Autodesk Inventor part; units mm, degrees
ref_plane "YZ Plane" through (0, 0, 0) normal (1, 0, 0) x (0, 1, 0)
ref_plane "XZ Plane" through (0, 0, 0) normal (0, 1, 0) x (-1, 0, 0)
ref_plane "XY Plane" through (0, 0, 0) normal (0, 0, 1) x (1, 0, 0)
ref_plane "Work Plane1" through (0, 0, 0) normal (0, 0, 1) x (1, 0, 0)
sketch "Sketch1" plane through (0, 0, 0) normal (0, 0, 1) x (1, 0, 0)
  line L0 (10.1591, -5.9453) -> (35.8591, -5.9453)
  line L1 (35.8591, -5.9453) -> (35.8591, -11.7453)
  line L2 (35.8591, -11.7453) -> (10.1591, -11.7453)
  line L3 (10.1591, -11.7453) -> (10.1591, -5.9453)
  point P0 (0, 0)
  dimension "d0" = 25.7
  dimension "d2" = 5.8
extrude "Extrusion1" add sketch "Sketch1" along normal blind 13.2
chamfer "Chamfer1" distance 9.2 angle 45 1 edges at (10.1591, -8.8453, 13.2)
sketch "Sketch2" plane through (35.8591, -11.7453, 0) normal (1, 0, 0) x (0, 0, -1)
  line L0 (0, 5.8) -> (0, 0)
  line L1 (0, 5.8) -> (-13.2, 5.8)
  line L2 (-13.2, 0) -> (-13.2, 5.8)
  line L3 (0, 0) -> (-13.2, 0)
  line L4 (-12.8, 5.4) -> (-0.4, 5.4)
  line L5 (-0.4, 5.4) -> (-0.4, 0.4)
  line L6 (-0.4, 0.4) -> (-12.8, 0.4)
  line L7 (-12.8, 0.4) -> (-12.8, 5.4)
  point P0 (0, 11.7453)
  dimension "d8" = 0.4
extrude "Extrusion2" cut sketch "Sketch2" against normal blind 16 contours L4 L5 L6 L7
sketch "Sketch3" plane through (19.8591, -11.7453, 0) normal (1, 0, 0) x (0, 0, -1)
  line L0 (-12.8, 5.4) -> (-0.4, 5.4)
  line L1 (-12.8, 0.4) -> (-12.8, 5.4)
  line L2 (-0.4, 5.4) -> (-0.4, 0.4)
  line L3 (-12.4, 5) -> (-0.8, 5)
  line L4 (-0.8, 5) -> (-0.8, 3.6)
  line L5 (-0.8, 3.6) -> (-12.4, 3.6)
  line L6 (-12.4, 3.6) -> (-12.4, 5)
  point P0 (0, 11.7453)
  dimension "d11" = 0.4
  dimension "d12" = 0.4
  dimension "d13" = 0.4
  dimension "d14" = 1.4
extrude "Extrusion3" add sketch "Sketch3" along normal blind 16
properties part number "nanopc_t4_usb3"
The model under review builds one solid part; all positions refer to its coordinate system, in mm. A direction names the side the tool comes from. Round coordinates to 2 decimals unless told otherwise and drop trailing zeros. Order: outer loops, then holes, each group sorted by start corner. A loop starts at its lowest first (then second) coordinate and runs counter-clockwise, first axis right, second up. Notation, with made-up numbers: (-36.75, 72.5) -> (13.25, 72.5) arc R30 cw to (13.25, 95.5) -> close; hole circle Ø10 at (6, -25.5). An arc over 180 degrees is marked (long way). Use CSV: the item, a comma, the result in double quotes. Start each with the question number.
(1) Consider section A-A on x = 34.25. Write out the cut boundary in (y, z), and give its area (3 significant figures).
(2) Mouldability with a two-part tool opening along Z and no side actions: class faces 1 (the face through (23, -5.945, 7)), 2 (the face through (19.859, -9, 7)), 3 (the face through (27, -9, 13.2)), 4 (the face through (28, -6.745, 7)) as pulls with the +Z half, pulls with the -Z half, needs draft (parallel to the pull), parting line crosses it, or undercut.
(3) Consider section D-D on y = -7.35. Write out the cut boundary in (x, z).
(4) Wall thickness on probe 1 along Y at (x, z) = (29.75, 11.5); probe 2 along Y at (x, z) = (24, 0.75); probe 3 along Z at (x, y) = (26.5, -11.15): over which ranges is each line inside the solid? List them lowest first. Write a range as from..to.
(5) Consider section B-B on y = -10.3. Write out the cut boundary in (x, z), and give its area (3 significant figures).
(6) Consider section C-C on z = 3.5. Write out the cut boundary in (x, y).
(7) Tool access review of faces 5 (the face through (23, -9, 0)), 6 (the face through (28, -7, 12.4)): name each direction out of +Z, -Z, +X, -X, +Y, -Y from which nothing blocks a thin tool from reaching the whole face with its end or side.
Responses:
1,outline,"(-11.75, 0) -> (-5.95, 0) -> (-5.95, 13.2) -> (-11.75, 13.2) -> close; (-8.15, 0.8) -> (-6.75, 0.8) -> (-6.75, 12.4) -> (-8.15, 12.4) -> close; hole (-11.35, 0.4) -> (-6.35, 0.4) -> (-6.35, 12.8) -> (-11.35, 12.8) -> close"
1,area,"30.8 mm²"
2,face 1,"needs draft"
2,face 2,"undercut"
2,face 3,"pulls with the +Z half"
2,face 4,"undercut"
3,outline,"(10.16, 0) -> (35.86, 0) -> (35.86, 0.4) -> (19.86, 0.4) -> (19.86, 0.8) -> (35.86, 0.8) -> (35.86, 12.4) -> (19.86, 12.4) -> (19.86, 12.8) -> (35.86, 12.8) -> (35.86, 13.2) -> (19.36, 13.2) -> (10.16, 4) -> close"
4,probe 1,"-11.75..-11.35, -8.15..-6.75, -6.35..-5.95"
4,probe 2,"-11.75..-11.35, -6.35..-5.95"
4,probe 3,"0..0.4, 12.8..13.2"
5,outline,"(10.16, 0) -> (35.86, 0) -> (35.86, 0.4) -> (19.86, 0.4) -> (19.86, 12.8) -> (35.86, 12.8) -> (35.86, 13.2) -> (19.36, 13.2) -> (10.16, 4) -> close"
5,area,"98.5 mm²"
6,outline,"(10.16, -11.75) -> (35.86, -11.75) -> (35.86, -11.35) -> (19.86, -11.35) -> (19.86, -8.15) -> (35.86, -8.15) -> (35.86, -6.75) -> (19.86, -6.75) -> (19.86, -6.35) -> (35.86, -6.35) -> (35.86, -5.95) -> (10.16, -5.95) -> close"
7,face 5,"-Z, +X, -X, +Y, -Y"
7,face 6,"+X"
